from build123d import *

# Parameters (mm, degrees)
F1_DEPTH    = 25
F2_DEPTH    = 1
F4_DEPTH    = 47.5
F5_R        = 3.1384776311
F6_T1_DEPTH = 41.8994949366


# Not quite as in the source:
# - a fillet or chamfer that OpenCascade refuses, or shapes differently, is made with other operations: its cross-section is extruded or revolved along the edge and cut away or added


with BuildPart() as f1:
    # F0 (on Right) → F1 (new body)
    with BuildSketch(Plane.YZ):
        Polygon((0, 43.8), (-29, 43.8), (-29, 41.8), (-4, 41.8), (-4, 2), (-29, 2), (-29, 0), (0, 0), align=None)
    extrude(amount=F1_DEPTH)

    # F2 (add): a face of the model
    f2_faces = [f1.faces().sort_by_distance(p)[0] for p in [
        (12.5, -4, 21.9),
    ]]
    extrude(f2_faces, amount=F2_DEPTH)

    # F3 (on face) → F4 (cut)
    with BuildSketch(Plane.XY.offset(43.8)):
        with BuildLine():
            Line((12.5, -3.075), (14.375, -3.075))
            ThreePointArc((14.375, -3.075), (12.5, -1.2), (10.625, -3.075))
            Line((10.625, -3.075), (12.5, -3.075))
        make_face()
        with BuildLine():
            Line((14.375, -29), (14.375, -3.075))
            ThreePointArc((14.375, -3.075), (12.5, -4.95), (10.625, -3.075))
            Line((10.625, -3.075), (10.625, -29))
            Line((10.625, -29), (14.375, -29))
        make_face()
        with BuildLine():
            ThreePointArc((10.625, -3.075), (12.5, -4.95), (14.375, -3.075))
            Line((14.375, -3.075), (12.5, -3.075))
            Line((12.5, -3.075), (10.625, -3.075))
        make_face()
    extrude(amount=-F4_DEPTH, mode=Mode.SUBTRACT)

    # F5
    f5_edges = [f1.edges().sort_by_distance(p)[0] for p in [
        (0, -29, 42.8),
        (10.625, -29, 42.8),
        (14.375, -29, 42.8),
        (25, -29, 42.8),
        (25, -29, 1),
        (14.375, -29, 1),
        (10.625, -29, 1),
        (0, -29, 1),
    ]]
    fillet(f5_edges, radius=F5_R)

    # F6: fillet of radius 3.3798989873 on 2 edges, made by hand

    # F6_s2 → F6_t1 (cut)
    with BuildSketch(Plane.YZ.offset(-8.4497474683)):
        with BuildLine():
            ThreePointArc((-3.3798989873, 43.8), (-0.9899494937, 42.8100505063), (0, 40.4201010127))
            Line((0, 40.4201010127), (0, 43.8))
            Line((0, 43.8), (-3.3798989873, 43.8))
        make_face()
        with BuildLine():
            ThreePointArc((0, 3.3798989873), (-0.9899494937, 0.9899494937), (-3.3798989873, 0))
            Line((-3.3798989873, 0), (0, 0))
            Line((0, 0), (0, 3.3798989873))
        make_face()
    extrude(amount=F6_T1_DEPTH, mode=Mode.SUBTRACT)


solid = f1.part
Could you check a few things on this model? Use its own coordinates, in mm. A direction names the side the tool comes from. Coordinates: 2 decimals unless noted, no trailing zeros. Order: outer loops, then holes, each group sorted by start corner. A loop starts at its lowest first (then second) coordinate and runs counter-clockwise, first axis right, second up.
Q1. Please list where these lines run through material, in increasing order: L1, parallel to Z at x = 1.5, y = -15; L2, parallel to X at y = -4.25, z = 13 (3 decimals); L3, parallel to Y at x = 24, z = 15.
Q2. Suppose I cut it at A-A on y = -15.5. Please give me the cut outline in (x, z) (3 decimals).
Q3. Suppose I cut it at D-D on x = 12.5. Please give me the cut outline in (y, z).
Q4. Thinking about a two-plate mould opening in Z: for faces 4 (the flat face through (5, -5, 22)), 5 (the flat face through (5, -16, 43.8)), 6 (the flat face through (20, -29, 1)), which applies, released by +Z, released by -Z, zero draft, split by the parting line, or undercut?
Q5. Will this pin go through, and if not, where does the flat tip stop? pin 1 (3 mm diameter, centred on x = 17.5, z = 11, fed in from -Y).
Q6. Which directions (+Z, -Z, +X, -X, +Y, -Y) give clear straight access to the entire face, cutting with the end or side of a thin tool? Please do faces 1 (the flat face through (5, -16, 0)), 2 (the flat face through (5, -17, 41.8)), 3 (the cylindrical face through (9.681, -28.105, 42.786)).
Q7. Suppose I cut it at B-B on z = 39. Please give me the cut outline in (x, y) (3 decimals), and give its area (3 significant figures).
Q8. Suppose I cut it at C-C on x = 18.75. Please give me the cut outline in (y, z), and give its area (3 significant figures).
Answer:
1. L1: z = 0 to 2, 41.8 to 43.8
1. L2: x = 0 to 10.625, 14.375 to 25
1. L3: y = -5 to 0
2. outline: (0, 0) - (10.625, 0) - (10.625, 2) - (0, 2) - close; (0, 41.8) - (10.625, 41.8) - (10.625, 43.8) - (0, 43.8) - close; (14.375, 0) - (25, 0) - (25, 2) - (14.375, 2) - close; (14.375, 41.8) - (25, 41.8) - (25, 43.8) - (14.375, 43.8) - close
3. outline: (-1.2, 0.8) arc R3.38 ccw to (0, 3.38) - (0, 40.42) arc R3.38 ccw to (-1.2, 43) - close
4. face 4: undercut
4. face 5: released by +Z
4. face 6: zero draft
5. pin 1: stops at y = -5
6. face 1: -Z, +X, -X, +Y, -Y
6. face 2: +X, -X, -Y
6. face 3: +Z, -Z, -Y
7. outline: (0, -5) - (10.625, -5) - (10.625, -3.075) arc R1.875 cw to (14.375, -3.075) - (14.375, -5) - (25, -5) - (25, 0) - (0, 0) - close
7. area: 112 mm2
8. outline: (-29, 0) - (-3.38, 0) arc R3.38 ccw to (0, 3.38) - (0, 40.42) arc R3.38 ccw to (-3.38, 43.8) - (-29, 43.8) - (-29, 41.8) - (-5, 41.8) - (-5, 2) - (-29, 2) - close
8. area: 310 mm2
